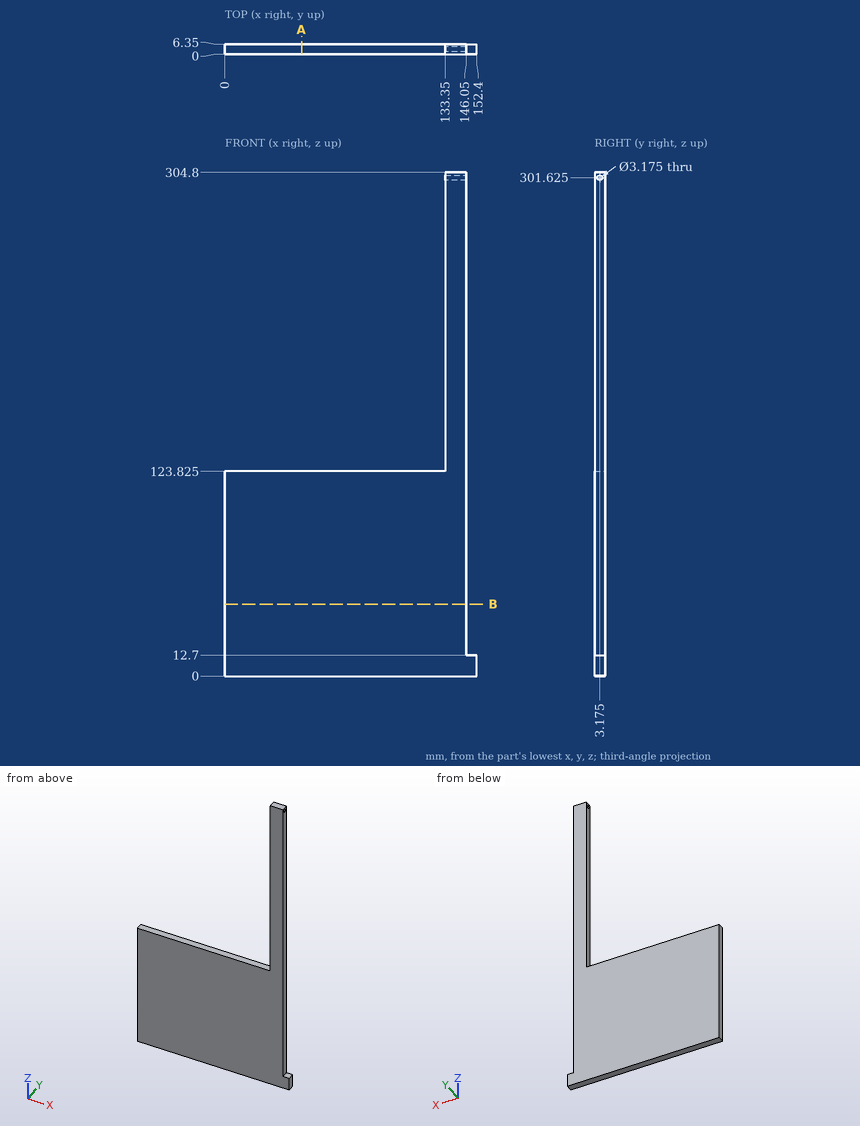
Geometry check sheet. Reference: drawing and pictorial views, mm from the part's lowest x, y, z. Round coordinates to 2 decimals unless told otherwise and drop trailing zeros. Loops run counter-clockwise (first coordinate to the right, second up) from the corner with the lowest first, then second, coordinate; pieces in that order, holes last. Notation, with made-up numbers: (8.5, 3.5) - (19.5, 3.5) arc R10 cw to (19.5, 16.5) - close; hole circle Ø1 at (16.5, 9.5). An arc over 180 degrees is marked (long way). Answer in a Markdown table with one row per item. Add a question column.
Q1. Section check B-B on z = 43.5. Enter the section's corners in (x, y).
Q2. Material ranges on line 1 (X direction, y = 4.25, z = 275.5); line 2 (X direction, y = 5.5, z = 25); line 3 (Z direction, x = 115.5, y = 0.5) (3 decimals), recorded low to high.
Q3. Gauge pin test, flat ends, axial feed: pin 1 (3 mm diameter, centred on x = 85.5, y = 4.5, fed in from +Z) (3 decimals); pin 2 (3 mm diameter, centred on x = 150.5, y = 3, fed in from +Z); pin 3 (3 mm diameter, centred on y = 3.5, z = 138, fed in from -X). Record the tip position at first contact, or that the pin passes through.
Q4. Section check A-A on x = 46.5. Enter the section's corners in (y, z) (3 decimals), plus the area to 3 significant figures.
Found:
| question | item | result |
|---|---|---|
| 1 | outline | (0, 0) - (146.05, 0) - (146.05, 6.35) - (0, 6.35) - close |
| 2 | line 1 | x = 133.35 to 146.05 |
| 2 | line 2 | x = 0 to 146.05 |
| 2 | line 3 | z = 0 to 123.825 |
| 3 | pin 1 | stops at z = 123.825 |
| 3 | pin 2 | stops at z = 12.7 |
| 3 | pin 3 | stops at x = 133.35 |
| 4 | outline | (0, 0) - (6.35, 0) - (6.35, 123.825) - (0, 123.825) - close |
| 4 | area | 786 mm² |
